from build123d import *

# Parameters (mm, degrees)
F1_DEPTH = 3.1
F3_W     = 8.5598
F3_H     = 9.975209
F4_DEPTH = 25.4


with BuildPart() as f1:
    # F0 (on Front) → F1 (new body)
    with BuildSketch(Plane.XZ):
        Polygon((-351.025, -37.88251), (-581.025, -37.88251), (-581.025, -118.84501), (-327.025, -118.84501), (-189.790466, -37.904931), (0, -37.904931), (0, 9.720069), (-223.572938, 9.720069), align=None)
    extrude(amount=F1_DEPTH)

    # F2: F1 across plane


with BuildPart() as f1_1:
    add(f1.part)
    add(f1.part.mirror(Plane.YZ))

    # F3 (on face) → F4 (cut)
    with BuildSketch(Plane.XZ.offset(3.1)):
        with Locations((401.249896, -53.270142)):
            Rectangle(F3_W, F3_H)
        with Locations((-401.249896, -53.270142)):
            Rectangle(F3_W, F3_H)
    extrude(amount=-F4_DEPTH, mode=Mode.SUBTRACT)


solid = f1_1.part
Could you check a few things on this model? Use its own coordinates, in mm. A direction names the side the tool comes from. Give positions to 0.01 mm unless a question says otherwise; leave off trailing zeros. Order: outer loops, then holes, each group sorted by start corner. A loop starts at its lowest first (then second) coordinate and runs counter-clockwise, first axis right, second up.
1. Suppose I cut it at A-A (y = -1.85). Write out the boundary of the cut face in (x, z) (3 decimals).
Answers below:
outline: (-581.025, -118.845) - (-327.025, -118.845) - (-189.79, -37.905) - (189.79, -37.905) - (327.025, -118.845) - (581.025, -118.845) - (581.025, -37.883) - (351.025, -37.883) - (223.573, 9.72) - (-223.573, 9.72) - (-351.025, -37.883) - (-581.025, -37.883) - close; hole (-405.53, -58.258) - (-396.97, -58.258) - (-396.97, -48.283) - (-405.53, -48.283) - close; hole (396.97, -58.258) - (405.53, -58.258) - (405.53, -48.283) - (396.97, -48.283) - close
2. For pin 1 (1.6 mm diameter, centred on x = 51.5, y = -1.5, fed in from -Z); pin 2 (0.9 mm diameter, centred on x = 458.5, y = -2, fed in from +Z), each with a flat end and sliding along its axis, tell me the tip position at first contact or that it passes through.
Answers below:
pin 1: stops at z = -37.9
pin 2: stops at z = -37.88
3. Suppose I cut it at D-D (z = -25). Write out the boundary of the cut face in (x, y).
Answers below:
outline: (-316.53, -3.1) - (316.53, -3.1) - (316.53, 0) - (-316.53, 0) - close
4. I need wall thicknesses on L1, parallel to Z at x = -410, y = -2.85; L2, parallel to Z at x = 75, y = -1; L3, parallel to X at y = -1.45, z = -80 (3 decimals). Which ranges of each line are inside material? Lowest first, please.
Answers below:
L1: z = -118.85 to -37.88
L2: z = -37.9 to 9.72
L3: x = -581.025 to -261.163, 261.163 to 581.025
5. Which directions (+Z, -Z, +X, -X, +Y, -Y) give clear straight access to the entire face, cutting with the end or side of a thin tool? Please do faces 1 (the flat face through (-259.368, -1.528, -78.942)), 2 (the flat face through (-286.41, -1.53, -13.75)).
Answers below:
face 1: -Z, +Y, -Y
face 2: +Z, -X, +Y, -Y
6. Thinking about a two-plate mould opening in X: for faces 3 (the flat face through (259.368, -1.528, -78.942)), 4 (the flat face through (8, -3.1, -25)), 5 (the flat face through (286.41, -1.53, -13.75)), which applies, +X half, -X half, draft (parallel to the pull), parting line (faces both ways), or undercut?
Answers below:
face 3: undercut
face 4: draft
face 5: +X half
7. Suppose I cut it at C-C (x = -479.5). Write out the boundary of the cut face in (y, z).
Answers below:
outline: (-3.1, -118.85) - (0, -118.85) - (0, -37.88) - (-3.1, -37.88) - close
8. Suppose I cut it at B-B (z = -79). Write out the boundary of the cut face in (x, y) (3 decimals), plus the area to 3 significant figures.
Answers below:
outline: (-581.025, -3.1) - (-259.467, -3.1) - (-259.467, 0) - (-581.025, 0) - close; (259.467, -3.1) - (581.025, -3.1) - (581.025, 0) - (259.467, 0) - close
area: 1,990 mm2
